Design review of the part built by this model. Coordinates are the model's own, in mm. Face numbers are marked on the shaded views. A direction names the side the tool comes from. Give positions to 0.01 mm unless a question says otherwise; leave off trailing zeros. Answer as CSV lines item,"result".
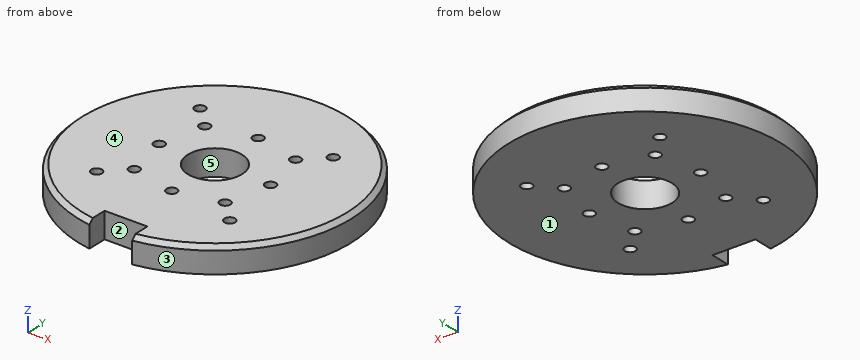
from build123d import *

# Parameters (mm, degrees)
SKETCH_1_R          = 31.75
EXTRUDE_1_DEPTH     = 6
SKETCH_2_W          = 10
SKETCH_2_H          = 10
CUT_EXTRUDE_1_DEPTH = 7
M3X0_52_D           = 2.5
M3X0_51_D           = 2.5
SKETCH_8_R          = 6.3
CUT_EXTRUDE_2_DEPTH = 7
CHAMFER_1_SIZE      = 1


with BuildPart() as part:
    # Эскиз1 → Бобышка-Вытянуть1 (new body)
    with BuildSketch(Plane.XY):
        Circle(SKETCH_1_R)
    extrude(amount=EXTRUDE_1_DEPTH)

    # Эскиз2 → Вырез-Вытянуть1 (cut, through all)
    with BuildSketch(Plane.XY.offset(6)):
        with Locations((0, -31.75)):
            Rectangle(SKETCH_2_W, SKETCH_2_H)
    extrude(amount=-CUT_EXTRUDE_1_DEPTH, mode=Mode.SUBTRACT)

    # Отверстие обработанное метчиком M3x0.52 (through all)
    with Locations(Plane.XY.offset(6)):
        with Locations((0, 13), (13, 0), (-13, 0), (0, -13)):
            Hole(M3X0_52_D / 2)

    # Отверстие обработанное метчиком M3x0.51 (through all)
    with Locations(Plane.XY.offset(6)):
        with Locations((-15.556349186, 15.556349186), (-15.556349186, -15.556349186), (15.556349186, -15.556349186), (15.556349186, 15.556349186), (10.606601718, 10.606601718), (-10.606601718, 10.606601718), (-10.606601718, -10.606601718), (10.606601718, -10.606601718)):
            Hole(M3X0_51_D / 2)

    # Эскиз8 → Вырез-Вытянуть2 (cut, through all)
    with BuildSketch(Plane.XY.offset(6)):
        Circle(SKETCH_8_R)
    extrude(amount=-CUT_EXTRUDE_2_DEPTH, mode=Mode.SUBTRACT)

    # Фаска1
    chamfer_1_edges = [part.edges().sort_by_distance(p)[0] for p in [
        (0, 31.75, 6),
    ]]
    chamfer(chamfer_1_edges, length=CHAMFER_1_SIZE)


solid = part.part
Q1. For the marked faces 1 and 2, list the 3-axis set-ups (+Z, -Z, +X, -X, +Y, -Y) from which the entire face can be reached by the end or side of a thin tool; tool diameter is ignored.
Filled sheet:
face 1,"-Z, +X, -X, +Y, -Y"
face 2,"+Z, -Z, -Y"
Q2. We need section A-A, the plane z = 4. State how many separate pieces and enclosed holes the cut face has, and give its area (3 significant figures).
Filled sheet:
separate pieces,"1"
enclosed holes,"13"
area,"2,930 mm^2"
Q3. To check wall thickness, follow probe 1 along Y at (x, z) = (0, 4); probe 2 along Y at (x, z) = (-16.5, 1.5); probe 3 along X at (y, z) = (14, 2.25). State the ranges of each line that lie inside material, in increasing order. Write a range as from..to.
Filled sheet:
probe 1,"y = -26.75..-14.25, -11.75..-6.3, 6.3..11.75, 14.25..31.75"
probe 2,"y = -27.13..-16.38, -14.74..14.74, 16.38..27.13"
probe 3,"x = -28.5..-0.75, 0.75..28.5"
Q4. The part is to be moulded in two halves that separate along Y. For the marked faces 3, 4 and 5, say which applies: pulls with the +Y half, pulls with the -Y half, needs draft (parallel to the pull), parting line crosses it, or undercut.
Filled sheet:
face 3,"parting line crosses it"
face 4,"needs draft"
face 5,"undercut"
Q5. Clearance check with a flat-ended pin moving along its axis: pin 1 Ø2.5 at (y, z) = (-28, 3) entering from -X. State where the tip first meets the part, or that it passes through.
Filled sheet:
pin 1,"stops at x = -17.1"
